Input: part model. Units: mm. Frame: model coordinates. Give positions to 0.01 mm unless a question says otherwise; leave off trailing zeros. Write each loop counter-clockwise with the first axis right and the second up, starting at its lowest first coordinate (ties: lowest second). Pieces come first, ordered by that corner, then holes. Notation, with made-up numbers: (21.5, 84) - (32.5, 84) arc R10 ccw to (32.5, 88) - close; hole circle Ø8 at (-9.75, 17.25). An arc over 180 degrees is marked (long way). Use a Markdown table: item, result. Add a question column.
1. Material intervals for probe 1 along Z at (x, y) = (2.5, 0); probe 2 along Y at (x, z) = (2, -5.5); probe 3 along Z at (x, y) = (2.75, 20), sorted ascending.
2. Section query A-A, the plane x = 4.75. Count the separate pieces of the cut face and the enclosed holes in it, plus the area to 3 significant figures.
3. Section query B-B, the plane y = 10. Return loops of the section in (x, z), plus the area to 3 significant figures.
4. Mould query, pull axis Y, two halves, no side actions, for faces 1 (the cylindrical face through (3.13, 25.66, 23.23)), 2 (the cylindrical face through (3.131, -31.073, 0.101)), 3 (the flat face through (3, 0, -38.124)). Classes: released by +Y, released by -Y, zero draft, split by the parting line, or undercut.
5. Pin query (flat end, axial travel): pin 1 (6 mm diameter, centred on y = -17.57, z = -19.07, fed in from -X); pin 2 (1.5 mm diameter, centred on x = 1.5, y = -15.5, fed in from +Z). Return the tip coordinate at first contact, or that it passes through.
6. Section query C-C, the plane z = 20. Return loops of the section in (x, y).
```python
from build123d import *

# Parameters (mm, degrees)
F0_R     = 2.286
F0_R_2   = 6.35
F1_DEPTH = 6.35


# Not quite as in the source:
# - ends of sketch curves that miss each other by under 0.0002 mm in the source are joined


with BuildPart() as f1:
    # F0 (on Right) → F1 (new body)
    with BuildSketch(Plane.YZ):
        with BuildLine():
            Line((-35.36227718, -1.6545656172), (-35.36227718, -38.1239391863))
            Line((-35.36227718, -38.1239391863), (-17.5702907145, -38.1239391863))
            Line((-17.5702907145, -38.1239391863), (0.221695751, -38.1239391863))
            Line((0.221695751, -38.1239391863), (18.0136822164, -38.1239391863))
            Line((18.0136822164, -38.1239391863), (35.8056686819, -38.1239391863))
            Line((35.8056686819, -38.1239391863), (35.8056686819, -1.6545656172))
            ThreePointArc((35.8056686819, -1.6545656172), (25.3839554031, 23.5071029235), (0.22312282, 33.9308342683))
            Line((0.22312282, 33.9308342683), (0.2202686819, 33.9308343828))
            ThreePointArc((0.2202686819, 33.9308343828), (-24.9405639012, 23.5071029235), (-35.36227718, -1.6545656172))
        make_face()
        with Locations((-0.074788043, -28.7147061436)):
            Circle(F0_R, mode=Mode.SUBTRACT)
        with BuildLine():
            ThreePointArc((-15.1890407145, -19.0739391863), (-15.8864926918, -20.757737209), (-17.5702907145, -21.4551891863))
            ThreePointArc((-17.5702907145, -21.4551891863), (-19.2540887372, -17.3901411636), (-15.1890407145, -19.0739391863))
        make_face(mode=Mode.SUBTRACT)
        with BuildLine():
            ThreePointArc((20.3949322164, -19.0739391863), (19.6974802391, -20.757737209), (18.0136822164, -21.4551891863))
            ThreePointArc((18.0136822164, -21.4551891863), (16.3298841937, -17.3901411636), (20.3949322164, -19.0739391863))
        make_face(mode=Mode.SUBTRACT)
        with Locations((-28.7894941866, 0)):
            Circle(F0_R, mode=Mode.SUBTRACT)
        Circle(F0_R_2, mode=Mode.SUBTRACT)
        with Locations((-0.0747941866, 28.7147)):
            Circle(F0_R, mode=Mode.SUBTRACT)
        with Locations((28.639911957, -6.1436e-06)):
            Circle(F0_R, mode=Mode.SUBTRACT)
    extrude(amount=F1_DEPTH)


solid = f1.part
```
Result sheet:
| question | item | result |
|---|---|---|
| 1 | probe 1 | z = -38.12 to -31, -26.43 to -6.35, 6.35 to 26.43, 31 to 33.93 |
| 1 | probe 2 | y = -35.36 to -3.17, 3.17 to 35.81 |
| 1 | probe 3 | z = -38.12 to -20.39, -17.76 to 27.93 |
| 2 | separate pieces | 1 |
| 2 | enclosed holes | 7 |
| 2 | area | 4,360 mm² |
| 3 | outline | (0, -38.12) - (6.35, -38.12) - (6.35, 32.56) - (0, 32.56) - close |
| 3 | area | 449 mm² |
| 4 | face 1 | released by +Y |
| 4 | face 2 | undercut |
| 4 | face 3 | zero draft |
| 5 | pin 1 | stops at x = 0 |
| 5 | pin 2 | stops at z = 30.63 |
| 6 | outline | (0, -28.02) - (6.35, -28.02) - (6.35, 28.46) - (0, 28.46) - close |
